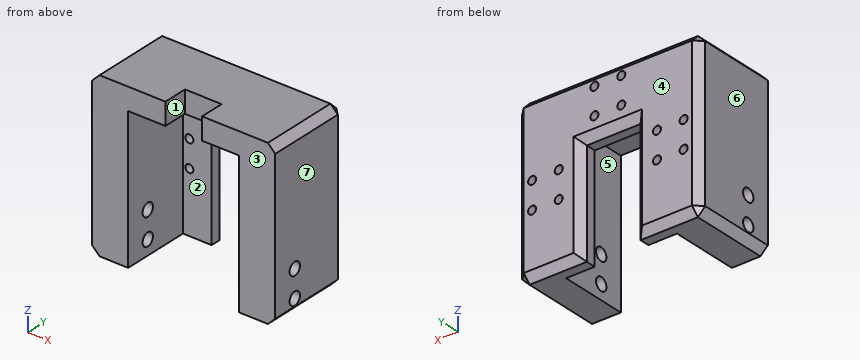
```python
from build123d import *

# Parameters (mm, degrees)
SKETCH1_W                 = 75
SKETCH1_H                 = 35
BOSS_EXTRUDE1_DEPTH       = 67
SKETCH2_W                 = 45.5
SKETCH2_H                 = 28
CUT_EXTRUDE1_DEPTH        = 58
SKETCH4_W                 = 15
SKETCH4_H                 = 10
CUT_EXTRUDE2_DEPTH        = 72.249561402
SKETCH5_W                 = 22
SKETCH5_H                 = 7
CUT_EXTRUDE3_DEPTH        = 43
F_3_0MM_DOWEL_HOLE1_D     = 3.3
F_3_0MM_DOWEL_HOLE1_DEPTH = 10
F_3_0MM_DOWEL_HOLE1_TIP   = 0.991420021
SKETCH8_R                 = 2.65
CUT_EXTRUDE4_DEPTH        = 103.079625783
CHAMFER1_SIZE             = 3


with BuildPart() as part:
    # Sketch1 → Boss-Extrude1 (new body)
    with BuildSketch(Plane.XY):
        Rectangle(SKETCH1_W, SKETCH1_H)
    extrude(amount=-BOSS_EXTRUDE1_DEPTH)

    # Sketch2 → Cut-Extrude1 (cut)
    with BuildSketch(Plane(origin=(0, 0, -67), x_dir=(-1, 0, 0), z_dir=(0, 0, -1))):
        with Locations((0, -3.5)):
            Rectangle(SKETCH2_W, SKETCH2_H)
    extrude(amount=-CUT_EXTRUDE1_DEPTH, mode=Mode.SUBTRACT)

    # Sketch4 → Cut-Extrude2 (cut, through all)
    with BuildSketch(Plane(origin=(0, 0, -9), x_dir=(-1, 0, 0), z_dir=(0, 0, -1))):
        with Locations((0, -12.5)):
            Rectangle(SKETCH4_W, SKETCH4_H)
    extrude(amount=-CUT_EXTRUDE2_DEPTH, mode=Mode.SUBTRACT)

    # Sketch5 → Cut-Extrude3 (cut)
    with BuildSketch(Plane(origin=(0, 0, -67), x_dir=(-1, 0, 0), z_dir=(0, 0, -1))):
        with Locations((0, 14)):
            Rectangle(SKETCH5_W, SKETCH5_H)
    extrude(amount=-CUT_EXTRUDE3_DEPTH, mode=Mode.SUBTRACT)

    # 3.0mm Dowel Hole1
    with Locations(Plane(origin=(0, 17.5, 0), x_dir=(1, 0, 0), z_dir=(0, 1, 0))):
        with Locations((-31.04375, 31), (-31.04375, 42), (-20.13125, 42), (-20.13125, 31), (-5.5, 16.36875), (5.5, 16.36875), (-5.5, 5.45625), (5.5, 5.45625), (31.04375, 42), (20.13125, 42), (31.04375, 31), (20.13125, 31)):
            Hole(F_3_0MM_DOWEL_HOLE1_D / 2, depth=F_3_0MM_DOWEL_HOLE1_DEPTH)
            with Locations((0, 0, -(F_3_0MM_DOWEL_HOLE1_DEPTH + F_3_0MM_DOWEL_HOLE1_TIP / 2))):  # 118° drill point
                Cone(0, F_3_0MM_DOWEL_HOLE1_D / 2, F_3_0MM_DOWEL_HOLE1_TIP, mode=Mode.SUBTRACT)

    # Sketch8 → Cut-Extrude4 (cut, through all)
    with BuildSketch(Plane.ZY.offset(37.5)):
        with Locations((-61, -7.5)):
            Circle(SKETCH8_R)
        with Locations((-50, -7.5)):
            Circle(SKETCH8_R)
    extrude(amount=-CUT_EXTRUDE4_DEPTH, mode=Mode.SUBTRACT)

    # Chamfer1
    chamfer1_edges = [part.edges().sort_by_distance(p)[0] for p in [
        (-37.5, 0, -67),
        (-24.25, 17.5, -67),
        (0, 17.5, -24),
        (11, 17.5, -45.5),
        (37.5, 0, -67),
        (-11, 17.5, -45.5),
        (-37.5, 0, 0),
        (0, 17.5, 0),
        (37.5, 0, 0),
        (-37.5, 17.5, -33.5),
        (37.5, 17.5, -33.5),
        (24.25, 17.5, -67),
    ]]
    chamfer(chamfer1_edges, length=CHAMFER1_SIZE)


solid = part.part
```
Input: part model. Units: mm. Frame: model coordinates. Face numbers are marked on the shaded views. A direction names the side the tool comes from. Give positions to 0.01 mm unless a question says otherwise; leave off trailing zeros. Write each loop counter-clockwise with the first axis right and the second up, starting at its lowest first coordinate (ties: lowest second). Pieces come first, ordered by that corner, then holes. Notation, with made-up numbers: (9.5, 82) - (47.5, 82) arc R15 cw to (47.5, 101) - close; hole circle Ø7 at (-9, 51). An arc over 180 degrees is marked (long way). Write item = value, one per line. Start each with the question number.
1. Section query C-C, the plane x = -12.5. Output: boundary loops of the cut face in (y, z).
2. Mould query, pull axis X, two halves, no side actions, for the marked faces 4, 5, 6 and 7. Classes: released by +X, released by -X, zero draft, split by the parting line, or undercut.
3. Section query B-B, the plane z = -61. Output: boundary loops of the cut face in (x, y), then the cut area to 3 significant figures.
4. Access query for the marked faces 1, 2 and 3. Directions: +Z, -Z, +X, -X, +Y, -Y. A direction counts if a zero-diameter tool reaches every point of the face in a straight line with its end or side. Return the directions, or none.
5. Ray query, L1, parallel to Z at x = 20, y = 13; L2, parallel to X at y = 14, z = -31; L3, parallel to X at y = -15, z = -49. Return the intervals inside material, ascending.
6. First-contact query: pin 1 Ø4 at (y, z) = (-7.5, -61) entering from +X; pin 2 Ø12 at (x, y) = (-4.5, 5.5) entering from -Z; pin 3 Ø2.5 at (x, z) = (31.04, -31) entering from +Y; pin 4 Ø8 at (x, z) = (-8.5, -19) entering from -Y. Flat tips, straight axial feed; report the tip coordinate or a pass-through.
7. Section query D-D, the plane y = -2.5. Output: boundary loops of the cut face in (x, z).
8. Section query A-A, the plane z = -45.5. Output: boundary loops of the cut face in (x, y), then the cut area to 3 significant figures.
Check sheet entries:
q1.outline = (-17.5, -9) - (10.5, -9) - (10.5, -67) - (14.5, -67) - (16, -65.5) - (16, -22.5) - (17.5, -21) - (17.5, -3) - (14.5, 0) - (-17.5, 0) - close
q2.face_4 = zero draft
q2.face_5 = undercut
q2.face_6 = released by -X
q2.face_7 = released by +X
q3.outline = (-37.5, -17.5) - (-22.75, -17.5) - (-22.75, -10.15) - (-37.5, -10.15) - close; (-37.5, -4.85) - (-22.75, -4.85) - (-22.75, 10.5) - (-11, 10.5) - (-11, 14.5) - (-14, 17.5) - (-34.5, 17.5) - (-37.5, 14.5) - close; (11, 10.5) - (22.75, 10.5) - (22.75, -4.85) - (37.5, -4.85) - (37.5, 14.5) - (34.5, 17.5) - (14, 17.5) - (11, 14.5) - close; (22.75, -17.5) - (37.5, -17.5) - (37.5, -10.15) - (22.75, -10.15) - close
q3.area = 1,020 mm2
q4.face_1 = +Z, -Z, -Y
q4.face_2 = -Z, -Y
q4.face_3 = +Z, -Z, +X, -X, -Y
q5.L1 = -67 to -43.64, -40.36 to -32.64, -29.36 to 0
q5.L2 = -37.5 to -32.69, -29.39 to -21.78, -18.48 to -11, 11 to 18.48, 21.78 to 29.39, 32.69 to 37.5
q5.L3 = -37.5 to -22.75, 22.75 to 37.5
q6.pin_1 = through
q6.pin_2 = -24
q6.pin_3 = 7.26
q6.pin_4 = 10.5
q7.outline = (-37.5, -64) - (-34.5, -67) - (-22.75, -67) - (-22.75, -9) - (22.75, -9) - (22.75, -67) - (34.5, -67) - (37.5, -64) - (37.5, -3) - (34.5, 0) - (-34.5, 0) - (-37.5, -3) - close
q8.outline = (-37.5, -17.5) - (-22.75, -17.5) - (-22.75, 10.5) - (-11, 10.5) - (-11, 14.5) - (-14, 17.5) - (-34.5, 17.5) - (-37.5, 14.5) - close; (11, 10.5) - (22.75, 10.5) - (22.75, -17.5) - (37.5, -17.5) - (37.5, 14.5) - (34.5, 17.5) - (14, 17.5) - (11, 14.5) - close
q8.area = 1,180 mm2
